Source: CAD feature listing. Evaluate the final solid. Frame: model axes, mm. A direction names the side the tool comes from. Round coordinates to 2 decimals unless told otherwise and drop trailing zeros. Order: outer loops, then holes, each group sorted by start corner. A loop starts at its lowest first (then second) coordinate and runs counter-clockwise, first axis right, second up. Notation, with made-up numbers: M 28.25,85.25 L 61.25,85.25 A23 ccw 61.25,105.25 Z; hole C -21.75,62 d8. An arc over 180 degrees is marked long. Answer in a Markdown table with one row per item. Add a question column.
```python
from build123d import *

# Parameters (mm, degrees)
F0_R     = 11.15
F1_DEPTH = 10
F2_R     = 11.5
F2_R_2   = 10
F3_DEPTH = 1
F4_R     = 0.5
F5_R     = 0.25
F6_R     = 0.5


with BuildPart() as f1:
    # F0 (on Top) → F1 (new body)
    with BuildSketch(Plane.XY):
        with BuildLine():
            ThreePointArc((14.875, 1.9324531042), (13.6283962301, 6.2663239778), (11.15, 10.0338178178))
            ThreePointArc((11.15, 10.0338178178), (-15, 0), (11.15, -10.0338178178))
            Line((11.15, -10.0338178178), (11.15, -20))
            ThreePointArc((11.15, -20), (0.9717865316, -31.1075708837), (-10.9806064461, -21.936177181))
            Line((-10.9806064461, -21.936177181), (-14.7721162952, -22.604722665))
            ThreePointArc((-14.7721162952, -22.604722665), (1.3073361412, -34.9429204714), (15, -20))
            Line((15, -20), (15, -2.7271780287))
            ThreePointArc((15, -2.7271780287), (14.7553944092, -0.4022476555), (14.875, 1.9324531042))
        make_face()
        Circle(F0_R, mode=Mode.SUBTRACT)
        with BuildLine():
            ThreePointArc((15, 2.7271780287), (14.9321711045, 2.3306537331), (14.875, 1.9324531042))
            ThreePointArc((14.875, 1.9324531042), (14.9687173799, 0.9682458366), (15, 0))
            Line((15, 0), (15, 2.7271780287))
        make_face()
        with BuildLine():
            Line((11.15, 13), (11.15, 10.0338178178))
            ThreePointArc((11.15, 10.0338178178), (13.6283962301, 6.2663239778), (14.875, 1.9324531042))
            ThreePointArc((14.875, 1.9324531042), (14.9321711045, 2.3306537331), (15, 2.7271780287))
            Line((15, 2.7271780287), (15, 13))
            Line((15, 13), (11.15, 13))
        make_face()
        with BuildLine():
            Line((15, 2.7271780287), (15, 0))
            Line((15, 0), (15, -2.7271780287))
            ThreePointArc((15, -2.7271780287), (25.6773170696, -14.4365249887), (40.9, -10.0338178178))
            Line((40.9, -10.0338178178), (40.9, 0))
            Line((40.9, 0), (40.9, 10.0338178178))
            ThreePointArc((40.9, 10.0338178178), (25.6773170696, 14.4365249887), (15, 2.7271780287))
        make_face()
        with Locations((29.75, 0)):
            Circle(F0_R, mode=Mode.SUBTRACT)
        with BuildLine():
            ThreePointArc((15, 0), (14.9687173799, 0.9682458366), (14.875, 1.9324531042))
            ThreePointArc((14.875, 1.9324531042), (14.7553944092, -0.4022476555), (15, -2.7271780287))
            Line((15, -2.7271780287), (15, 0))
        make_face()
        with BuildLine():
            ThreePointArc((44.75, 0), (43.7544635742, 5.3735463151), (40.9, 10.0338178178))
            Line((40.9, 10.0338178178), (40.9, 0))
            Line((40.9, 0), (40.9, -10.0338178178))
            ThreePointArc((40.9, -10.0338178178), (43.7544635742, -5.3735463151), (44.75, 0))
        make_face()
        with BuildLine():
            Line((40.9, 13), (40.9, 10.0338178178))
            ThreePointArc((40.9, 10.0338178178), (43.7544635742, 5.3735463151), (44.75, 0))
            Line((44.75, 0), (44.75, 13))
            Line((44.75, 13), (40.9, 13))
        make_face()
        with BuildLine():
            ThreePointArc((44.75, 0), (43.7544635742, -5.3735463151), (40.9, -10.0338178178))
            Line((40.9, -10.0338178178), (40.9, -28.15))
            Line((40.9, -28.15), (44.75, -28.15))
            Line((44.75, -28.15), (44.75, 0))
        make_face()
        with BuildLine():
            Line((44.75, -28.15), (40.9, -28.15))
            ThreePointArc((40.9, -28.15), (47.1529831622, -34.9739336819), (54.4959331081, -29.339490017))
            Line((54.4959331081, -29.339490017), (50.704423259, -28.670944533))
            ThreePointArc((50.704423259, -28.670944533), (47.4885327718, -31.1385840943), (44.75, -28.15))
        make_face()
    extrude(amount=F1_DEPTH)

    # F2 (on Top) → F3 (join)
    with BuildSketch(Plane.XY):
        Circle(F2_R)
        Circle(F2_R_2, mode=Mode.SUBTRACT)
        with Locations((29.75, 0)):
            Circle(F2_R)
        with Locations((29.75, 0)):
            Circle(F2_R_2, mode=Mode.SUBTRACT)
    extrude(amount=F3_DEPTH)

    # F4
    f4_edges = [f1.edges().sort_by_distance(p)[0] for p in [
        (-10, 0, 1),
        (19.75, 0, 1),
    ]]
    fillet(f4_edges, radius=F4_R)

    # F5
    f5_edges = [f1.edges().sort_by_distance(p)[0] for p in [
        (15, -2.727178, 5),
        (15, 2.727178, 5),
        (11.15, 10.033818, 5),
        (40.9, 10.033818, 5),
        (11.15, -10.033818, 5),
        (40.9, -10.033818, 5),
    ]]
    fillet(f5_edges, radius=F5_R)

    # F6
    f6_edges = [f1.edges().sort_by_distance(p)[0] for p in [
        (-10.980606, -21.936177, 5),
        (-14.772116, -22.604723, 5),
        (11.15, 13, 5),
        (15, 13, 5),
        (40.9, 13, 5),
        (44.75, 13, 5),
        (54.495933, -29.33949, 5),
        (50.704423, -28.670945, 5),
    ]]
    fillet(f6_edges, radius=F6_R)


solid = f1.part
```
(1) Cut plane B-B (y = 0). Return loops of the section in (x, z), and give its area (3 significant figures).
(2) Cut plane C-C (x = 0). Return loops of the section in (y, z).
(3) Cut plane D-D (z = 9). Count the separate pieces of the cut face and the enclosed holes in it, and give its area (3 significant figures).
(4) Draft query along X for faces 4 (the face through (19, -10, 10)), 5 (the face through (1.437, -31.057, 4.93)), 6 (the face through (44.75, -8, 5)). Return one class per face: +X half, -X half, draft (parallel to the pull), parting line (faces both ways), or undercut.
(5) Pin query (flat end, axial travel): pin 1 (5 mm diameter, centred on x = 37.5, z = 6.5, fed in from +Y); pin 2 (2.5 mm diameter, centred on x = 43, z = 5.5, fed in from +Y); pin 3 (4 mm diameter, centred on y = 10.5, z = 3, fed in from +X). Return the tip coordinate at first contact, or that it passes through.
(6) Line query: line 1 (Y direction, x = 0, z = 0.1); line 2 (Y direction, x = 0, z = 4.25); line 3 (X direction, y = -19.5, z = 6.25). Output: solid intervals per line, ascending. Write a range as from..to.
(7) Cut plane A-A (x = 29.75). Return loops of the section in (y, z), and give its area (3 significant figures).
(8) Access query for faces 1 (the face through (40.9, 12, 5)), 2 (the face through (40.4, 3.3, 5.4)), 3 (the face through (40.9, -19, 5)). Directions: +Z, -Z, +X, -X, +Y, -Y. A direction counts if a zero-diameter tool reaches every point of the face in a straight line with its end or side. Return the directions, or none.
Answer list:
| question | item | result |
|---|---|---|
| 1 | outline | M -15,0 L -10,0 L -10,0.5 A0.5 ccw -10.5,1 L -11.15,1 L -11.15,10 L -15,10 Z; M 10,0 L 19.75,0 L 19.75,0.5 A0.5 ccw 19.25,1 L 18.6,1 L 18.6,10 L 11.15,10 L 11.15,1 L 10.5,1 A0.5 ccw 10,0.5 Z; M 39.75,0 L 44.75,0 L 44.75,10 L 40.9,10 L 40.9,1 L 40.25,1 A0.5 ccw 39.75,0.5 Z |
| 1 | area | 156 mm² |
| 2 | outline | M -35,0 L -31.15,0 L -31.15,10 L -35,10 Z; M -15,0 L -10,0 L -10,0.5 A0.5 ccw -10.5,1 L -11.15,1 L -11.15,10 L -15,10 Z; M 10,0 L 15,0 L 15,10 L 11.15,10 L 11.15,1 L 10.5,1 A0.5 ccw 10,0.5 Z |
| 3 | separate pieces | 1 |
| 3 | enclosed holes | 2 |
| 3 | area | 1,020 mm² |
| 4 | face 4 | draft |
| 4 | face 5 | undercut |
| 4 | face 6 | +X half |
| 5 | pin 1 | y = 14.05 |
| 5 | pin 2 | y = 13 |
| 5 | pin 3 | x = 44.75 |
| 6 | line 1 | -35..-31.15, -15..-10, 10..15 |
| 6 | line 2 | -35..-31.15, -15..-11.15, 11.15..15 |
| 6 | line 3 | 11.15..15, 40.9..44.75 |
| 7 | outline | M -15,0 L -10,0 L -10,0.5 A0.5 ccw -10.5,1 L -11.15,1 L -11.15,10 L -15,10 Z; M 10,0 L 15,0 L 15,10 L 11.15,10 L 11.15,1 L 10.5,1 A0.5 ccw 10,0.5 Z |
| 7 | area | 79.2 mm² |
| 8 | face 1 | +Z, -Z, +Y |
| 8 | face 2 | +Z |
| 8 | face 3 | +Z, -Z, -Y |
